Design review of the part built by this model. Coordinates are the model's own, in mm. Face numbers are marked on the shaded views. Coordinates: 2 decimals unless noted, no trailing zeros. Write each loop counter-clockwise with the first axis right and the second up, starting at its lowest first coordinate (ties: lowest second). Pieces come first, ordered by that corner, then holes. Notation, with made-up numbers: (2.25, 14.5) - (38.25, 14.5) arc R23 ccw to (38.25, 41.5) - close; hole circle Ø3 at (12.25, 38). An arc over 180 degrees is marked (long way). Use a Markdown table: item, result.
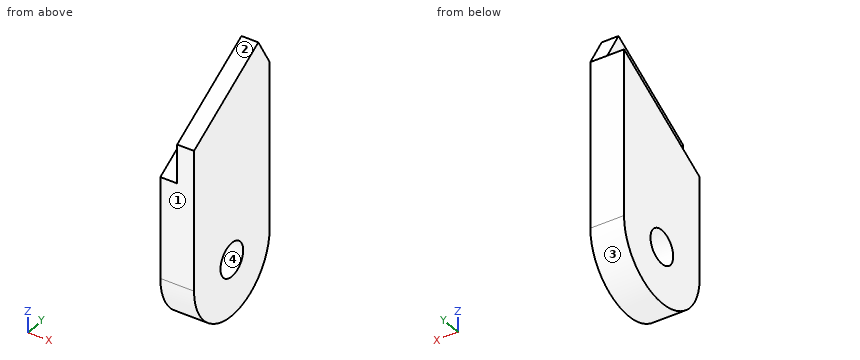
from build123d import *

# Parameters (mm, degrees)
SKETCH1_R           = 3
BOSS_EXTRUDE1_DEPTH = 6
CUT_EXTRUDE1_DEPTH  = 3


with BuildPart() as part:
    # Sketch1 → Boss-Extrude1 (new body)
    with BuildSketch(Plane(origin=(0, 0, 0), x_dir=(0, 0, -1), z_dir=(1, 0, 0))):
        with BuildLine():
            Line((-4.618802154, 20), (-9.814954576, 17))
            Line((-9.814954576, 17), (0, 0))
            Line((0, 0), (25, 0))
            ThreePointArc((25, 0), (35, 10), (25, 20))
            Line((25, 20), (-4.618802154, 20))
        make_face()
        with Locations((25, 10)):
            Circle(SKETCH1_R, mode=Mode.SUBTRACT)
    extrude(amount=BOSS_EXTRUDE1_DEPTH)

    # Sketch2 → Cut-Extrude1 (cut)
    with BuildSketch(Plane.ZY):
        Polygon((9.814954576, 17), (4.618802154, 20), (-6.92820323, 0), (0, 0), align=None)
    extrude(amount=-CUT_EXTRUDE1_DEPTH, mode=Mode.SUBTRACT)


solid = part.part
(1) Draft analysis for pull direction Z (two halves, no side actions). For the marked faces 1, 2, 3 and 4, state which applies: +Z half, -Z half, draft (parallel to the pull), parting line (faces both ways), or undercut.
Determined:
| item | result |
|---|---|
| face 1 | draft |
| face 2 | +Z half |
| face 3 | -Z half |
| face 4 | undercut |
(2) Take a section at D-D on z = 4. Write out the cut boundary in (x, y), and give its area (3 significant figures).
Determined:
| item | result |
|---|---|
| outline | (0, 18.93) - (3, 18.93) - (3, 6.93) - (6, 6.93) - (6, 20) - (0, 20) - close |
| area | 42.4 mm2 |
(3) For L1, parallel to Y at x = 1.9, z = -25; L2, parallel to X at y = 10.75, z = 3.5; L3, parallel to Z at x = 4.75, y = 14.75, list the stretches that pass through material, from the lowest coordinate up. Write a range as from..to.
Determined:
| item | result |
|---|---|
| L1 | 0..7, 13..20 |
| L2 | 3..6 |
| L3 | -33.8..8.52 |
(4) Take a section at B-B on y = 8.25. Write out the cut boundary in (x, z), and give its area (3 significant figures).
Determined:
| item | result |
|---|---|
| outline | (0, -34.85) - (6, -34.85) - (6, -27.44) - (0, -27.44) - close; (0, -22.56) - (6, -22.56) - (6, 4.76) - (3, 4.76) - (3, -2.17) - (0, -2.17) - close |
| area | 188 mm2 |
(5) Take a section at A-A on x = 2. Write out the cut boundary in (y, z), and give its area (3 significant figures).
Determined:
| item | result |
|---|---|
| outline | (0, -25) arc R10 ccw to (20, -25) - (20, 4.62) - (0, -6.93) - close; hole circle Ø6 at (10, -25) |
| area | 606 mm2 |
(6) Take a section at C-C on y = 2.25. Write out the cut boundary in (x, z), and give its area (3 significant figures).
Determined:
| item | result |
|---|---|
| outline | (0, -31.32) - (6, -31.32) - (6, 1.3) - (3, 1.3) - (3, -5.63) - (0, -5.63) - close |
| area | 175 mm2 |
(7) For pin 1 (3 mm diameter, centred on x = 3, z = -8, fed in from -Y); pin 2 (3 mm diameter, centred on x = 2.5, y = 10, fed in from +Z); pin 3 (1 mm diameter, centred on x = 4, z = 4.5, fed in from -Y), all flat-tipped, find the tip position at first contact; note any pin that passes through.
Determined:
| item | result |
|---|---|
| pin 1 | y = 0 |
| pin 2 | z = 6.59 |
| pin 3 | y = 6.93 |
